```python
from build123d import *

# Parameters (mm, degrees)
ESQUISSE1_W             = 8
ESQUISSE1_H             = 20
ESQUISSE1_R             = 1.55
BOSS_EXTRU_1_DEPTH      = 8
ESQUISSE2_R             = 1.55
ENL_V_MAT_EXTRU_1_DEPTH = 16.099668871
ESQUISSE3_R             = 1.9
ENL_V_MAT_EXTRU_2_DEPTH = 3
ENL_V_MAT_EXTRU_3_DEPTH = 5
CONG_1_R                = 2


with BuildPart() as part:
    # Esquisse1 → Boss.-Extru.1 (new body)
    with BuildSketch(Plane(origin=(0, 0, 0), x_dir=(0, 0, -1), z_dir=(1, 0, 0))):
        Rectangle(ESQUISSE1_W, ESQUISSE1_H)
        with Locations((0, 6)):
            Circle(ESQUISSE1_R, mode=Mode.SUBTRACT)
        with Locations(Location((0, -6, 0), (0, 0, 180))):
            Circle(ESQUISSE1_R, mode=Mode.SUBTRACT)
    extrude(amount=BOSS_EXTRU_1_DEPTH)

    # Esquisse2 → Enlèv. mat.-Extru.1 (cut, through all)
    with BuildSketch(Plane(origin=(0, 0, -4), x_dir=(-1, 0, 0), z_dir=(0, 0, -1))):
        with Locations((-4, 0)):
            Circle(ESQUISSE2_R)
    extrude(amount=-ENL_V_MAT_EXTRU_1_DEPTH, mode=Mode.SUBTRACT)

    # Esquisse3 → Enlèv. mat.-Extru.2 (cut)
    with BuildSketch(Plane(origin=(8, 0, 0), x_dir=(0, 0, -1), z_dir=(1, 0, 0))):
        with Locations((0, 6)):
            Circle(ESQUISSE3_R)
        with Locations((0, -6)):
            Circle(ESQUISSE3_R)
    extrude(amount=-ENL_V_MAT_EXTRU_2_DEPTH, mode=Mode.SUBTRACT)

    # Esquisse4 → Enlèv. mat.-Extru.3 (cut)
    with BuildSketch(Plane(origin=(0, 0, -4), x_dir=(-1, 0, 0), z_dir=(0, 0, -1))):
        Polygon((-5.58771324, 2.75), (-7.175426481, 0), (-5.58771324, -2.75), (-2.41228676, -2.75), (-0.824573519, 0), (-2.41228676, 2.75), align=None)
    extrude(amount=-ENL_V_MAT_EXTRU_3_DEPTH, mode=Mode.SUBTRACT)

    # Congé1
    cong_1_edges = [part.edges().sort_by_distance(p)[0] for p in [
        (4, -10, -4),
        (4, -10, 4),
        (4, 10, 4),
        (4, 10, -4),
    ]]
    fillet(cong_1_edges, radius=CONG_1_R)


solid = part.part
```
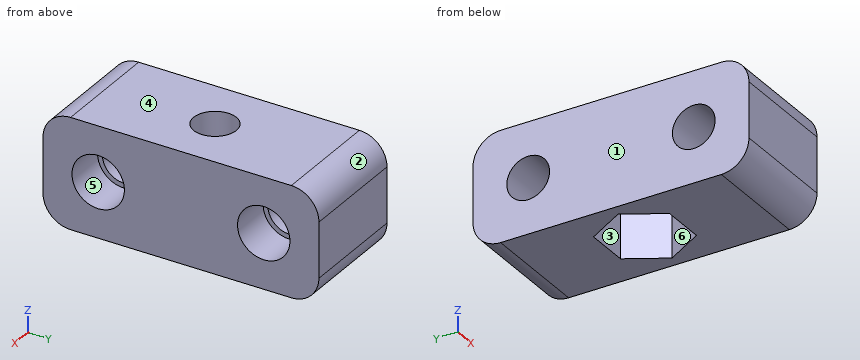
Could you check a few things on this model? Use its own coordinates, in mm. Face numbers are marked on the shaded views. A direction names the side the tool comes from. Round coordinates to 2 decimals unless told otherwise and drop trailing zeros. Write each loop counter-clockwise with the first axis right and the second up, starting at its lowest first coordinate (ties: lowest second). Pieces come first, ordered by that corner, then holes. Notation, with made-up numbers: M 33,67.5 L 41,67.5 A16 cw 41,96.5 Z; hole C 74,32.25 d6. An arc over 180 degrees is marked long. Answer in a Markdown table with one row per item. Add a question column.
Q1. Imagine slicing it at D-D (z = -3.5). Please give me the cut outline in (x, y), then the cut area to 3 significant figures.
Q2. If I drill on line 1 (Y direction, x = 4.75, z = 0); line 2 (Y direction, x = 6.9, z = 0); line 3 (Y direction, x = 4.5, z = -3.25), over which ranges is the centre line in solid material (lowest first)? Write a range as from..to.
Q3. Imagine slicing it at A-A (x = 4). Please give me the cut outline in (y, z).
Q4. If we mould it in two halves opening along X, with no side actions, what happens to the marked faces 1, 2 and 3? For each: +X half, -X half, draft (parallel to the pull), parting line (faces both ways), or undercut.
Q5. Imagine slicing it at B-B (z = 0). Please give me the cut outline in (x, y), then the cut area to 3 significant figures.
Q6. Imagine slicing it at C-C (y = 6). Please give me the cut outline in (x, z).
Q7. On a 3-axis mill with a long thin cutter (end or side, diameter ignored), from which of +Z, -Z, +X, -X, +Y, -Y can I reach the whole of each face in a straight line? I mean the marked faces 4, 5 and 6. Say none if no direction works.
Q8. Will these pins go through, and if not, where does the flat tip stop? pin 1 Ø1.1 at (y, z) = (5.5, -0.5) entering from +X; pin 2 Ø3.5 at (y, z) = (6, 0) entering from +X.
Values:
| question | item | result |
|---|---|---|
| 1 | outline | M 0,-9.32 L 8,-9.32 L 8,9.32 L 0,9.32 Z; hole M 0.82,0 L 2.41,-2.75 L 5.59,-2.75 L 7.18,0 L 5.59,2.75 L 2.41,2.75 Z |
| 1 | area | 123 mm^2 |
| 2 | line 1 | -10..-7.55, -4.45..-2.75, 2.75..4.45, 7.55..10 |
| 2 | line 2 | -10..-7.9, -4.1..-0.48, 0.48..4.1, 7.9..10 |
| 2 | line 3 | -9.56..-2.75, 2.75..9.56 |
| 3 | outline | M -10,-2 A2 ccw -8,-4 L -2.75,-4 L -2.75,1 L -1.55,1 L -1.55,4 L -8,4 A2 ccw -10,2 Z; M 1.55,1 L 2.75,1 L 2.75,-4 L 8,-4 A2 ccw 10,-2 L 10,2 A2 ccw 8,4 L 1.55,4 Z; hole C -6,0 d3.1; hole C 6,0 d3.1 |
| 4 | face 1 | -X half |
| 4 | face 2 | draft |
| 4 | face 3 | undercut |
| 5 | outline | M 0,-10 L 8,-10 L 8,-7.9 L 5,-7.9 L 5,-7.55 L 0,-7.55 Z; M 0,-4.45 L 5,-4.45 L 5,-4.1 L 8,-4.1 L 8,4.1 L 5,4.1 L 5,4.45 L 0,4.45 Z; M 0,7.55 L 5,7.55 L 5,7.9 L 8,7.9 L 8,10 L 0,10 Z; hole M 0.82,0 L 2.41,-2.75 L 5.59,-2.75 L 7.18,0 L 5.59,2.75 L 2.41,2.75 Z |
| 5 | area | 80.0 mm^2 |
| 6 | outline | M 0,-4 L 8,-4 L 8,-1.9 L 5,-1.9 L 5,-1.55 L 0,-1.55 Z; M 0,1.55 L 5,1.55 L 5,1.9 L 8,1.9 L 8,4 L 0,4 Z |
| 7 | face 4 | +Z, +X, -X, +Y, -Y |
| 7 | face 5 | +X |
| 7 | face 6 | -Z |
| 8 | pin 1 | through |
| 8 | pin 2 | x = 5 |
